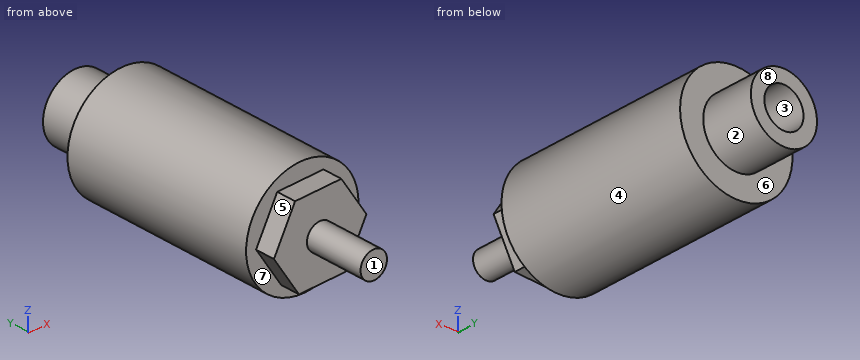
```python
from build123d import *

# Parameters (mm, degrees)
SKETCH1_W           = 8.5
SKETCH1_H           = 30
BOSS_EXTRUDE1_DEPTH = 3
SKETCH3_R           = 5
BOSS_EXTRUDE2_DEPTH = 8
SKETCH4_W           = 2
SKETCH4_H           = 9
HOLE1_D             = 5.917
HOLE1_DEPTH         = 14
HOLE1_TIP           = 1.777646141


with BuildPart() as part:
    # Sketch1 → Revolve1 (revolve)
    with BuildSketch(Plane.XY):
        with Locations((4.25, -15)):
            Rectangle(SKETCH1_W, SKETCH1_H)
    revolve(axis=Axis((0, 0, 0), (0, -1, 0)))

    # Sketch2 → Boss-Extrude1 (add)
    with BuildSketch(Plane.XZ.offset(30)):
        Polygon((-3.79267276, 5.883505191), (3.198928579, 6.226303554), (6.991601339, 0.342798363), (3.79267276, -5.883505191), (-3.198928579, -6.226303554), (-6.991601339, -0.342798363), align=None)
    extrude(amount=BOSS_EXTRUDE1_DEPTH)

    # Sketch3 → Boss-Extrude2 (add)
    with BuildSketch(Plane(origin=(0, 0, 0), x_dir=(-1, 0, 0), z_dir=(0, 1, 0))):
        Circle(SKETCH3_R)
    extrude(amount=BOSS_EXTRUDE2_DEPTH)

    # Sketch4 → Revolve2 (revolve)
    with BuildSketch(Plane.XY):
        with Locations((1, -37.5)):
            Rectangle(SKETCH4_W, SKETCH4_H)
    revolve(axis=Axis((0, -33, 0), (0, -1, 0)))

    # Hole1
    with Locations(Plane(origin=(0, 8, 0), x_dir=(1, 0, 0), z_dir=(0, 1, 0))):
        with Locations((0, 0)):
            Hole(HOLE1_D / 2, depth=HOLE1_DEPTH)
            with Locations((0, 0, -(HOLE1_DEPTH + HOLE1_TIP / 2))):  # 118° drill point
                Cone(0, HOLE1_D / 2, HOLE1_TIP, mode=Mode.SUBTRACT)


solid = part.part
```
Verification items for the finished model (mm, model axes). Face numbers are marked on the shaded views. A direction names the side the tool comes from. Give positions to 0.01 mm unless a question says otherwise; leave off trailing zeros. Write each loop counter-clockwise with the first axis right and the second up, starting at its lowest first coordinate (ties: lowest second). Pieces come first, ordered by that corner, then holes. Notation, with made-up numbers: (75, 80) - (115, 80) arc R16 cw to (115, 102) - close; hole circle Ø5 at (-3, 4.5). An arc over 180 degrees is marked (long way). Put each result on its own line as item: value.
Q1. Set-up check for the marked faces 4, 5, 6, 7 and 8: record each of +Z, -Z, +X, -X, +Y, -Y from which the full face is reachable in a straight line by a thin tool's end or side.
Result:
face 4: +Y, -Y
face 5: +Z, -X, -Y
face 6: +Y
face 7: -Y
face 8: +Z, -Z, +X, -X, +Y
Q2. Section check B-B on x = 6. Record the cut outline in (y, z), and give its area (3 significant figures).
Result:
outline: (-33, -1.59) - (-30, -1.59) - (-30, -6.02) - (0, -6.02) - (0, 6.02) - (-30, 6.02) - (-30, 1.88) - (-33, 1.88) - close
area: 372 mm2
Q3. Mould release check, pull along Z, two halves, no side actions. Record for the marked faces 1, 2 and 3: released by +Z, released by -Z, zero draft, split by the parting line, or undercut.
Result:
face 1: zero draft
face 2: split by the parting line
face 3: undercut
Q4. Section check A-A on y = -3.5. Record the cut outline in (x, z), and give its area (3 significant figures).
Result:
outline: circle Ø17 at (0, 0); hole circle Ø5.92 at (0, 0)
area: 199 mm2
Q5. Section check C-C on y = -36. Record the cut outline in (x, z).
Result:
outline: circle Ø4 at (0, 0)
Q6. Scan lines: probe 1 along Z at (x, y) = (0, 1); probe 2 along Z at (x, y) = (0, -2.25); probe 3 along Y at (x, z) = (0.5, -7.5). Record each from-to range of solid material in increasing order. Write a range as from..to.
Result:
probe 1: -5..-2.96, 2.96..5
probe 2: -8.5..-2.96, 2.96..8.5
probe 3: -30..0
Q7. Section check D-D on y = -14. Record the cut outline in (x, z), and give its area (3 significant figures).
Result:
outline: circle Ø17 at (0, 0)
area: 227 mm2
Q8. Depth check by flat-ended pin: P1, Ø5.5, axis at x = 0, z = 0, coming from the +Y side; P2, Ø8, axis at x = 5.5, y = -32.5, coming from the -Z side. Enter the tip coordinate at first touch or a pass-through.
Result:
P1: y = -6.13
P2: z = -8.16
